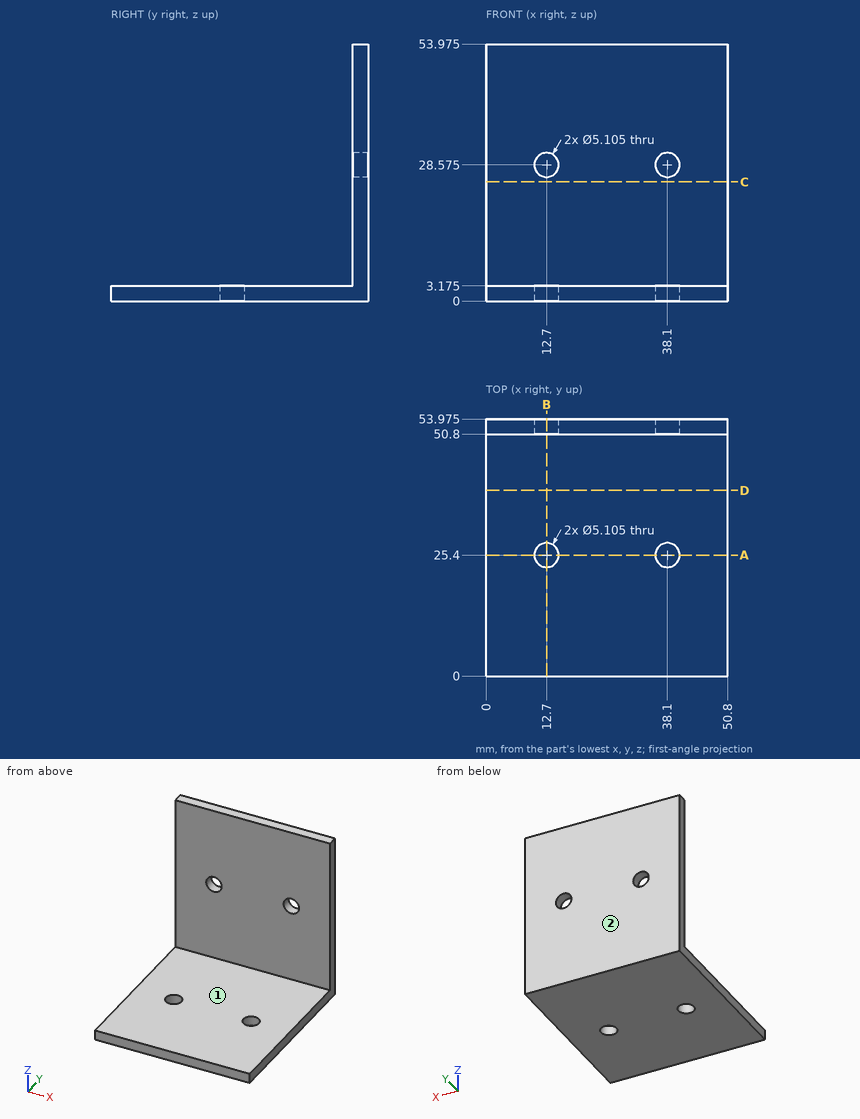
Input: dimensioned drawing with shaded views. Units: mm. Origin: part minimum x, y, z. A direction names the side the tool comes from. Round coordinates to 2 decimals unless told otherwise and drop trailing zeros. Order: outer loops, then holes, each group sorted by start corner. A loop starts at its lowest first (then second) coordinate and runs counter-clockwise, first axis right, second up. Notation, with made-up numbers: (24.5, -18.5) - (39.5, -18.5) arc R32 ccw to (39.5, 12.5) - close; hole circle Ø6 at (29, 48). An arc over 180 degrees is marked (long way). Answer as a JSON object with one key per item and string values. Group by question number.
(1) Pin query (flat end, axial travel): P1, Ø10, axis at x = 21.5, z = 27.5, coming from the -Y side. Return the tip coordinate at first contact, or that it passes through.
(2) Material intervals for probe 1 along Y at (x, z) = (38.1, 2.05) (1 decimal); probe 2 along Z at (x, y) = (38, 51) (1 decimal); probe 3 along Y at (x, z) = (24, 8) (1 decimal), sorted ascending. Write a range as from..to.
(3) Cut plane D-D (y = 39). Return loops of the section in (x, z) (1 decimal).
(4) Cut plane B-B (x = 12.7). Return loops of the section in (y, z) (1 decimal), then the cut area to 3 significant figures.
(5) Cut plane A-A (y = 25.4). Return loops of the section in (x, z) (1 decimal).
(6) Cut plane C-C (z = 25). Return loops of the section in (x, y) (1 decimal).
(7) Reachability of the marked faces 1 and 2 from +Z, -Z, +X, -X, +Y, -Y: full face, straight path, thin tool, end or side. Return the list, or none.
Here are the results:
{
 "1": {"P1": "stops at y = 50.8"},
 "2": {"probe 1": "y = 0..22.8, 28..54", "probe 2": "z = 0..26, 31.1..54", "probe 3": "y = 50.8..54"},
 "3": {"outline": "(0, 0) - (50.8, 0) - (50.8, 3.2) - (0, 3.2) - close"},
 "4": {"outline": "(0, 0) - (22.8, 0) - (22.8, 3.2) - (0, 3.2) - close; (28, 0) - (54, 0) - (54, 26) - (50.8, 26) - (50.8, 3.2) - (28, 3.2) - close; (50.8, 31.1) - (54, 31.1) - (54, 54) - (50.8, 54) - close", "area": "300 mm^2"},
 "5": {"outline": "(0, 0) - (10.1, 0) - (10.1, 3.2) - (0, 3.2) - close; (15.3, 0) - (35.5, 0) - (35.5, 3.2) - (15.3, 3.2) - close; (40.7, 0) - (50.8, 0) - (50.8, 3.2) - (40.7, 3.2) - close"},
 "6": {"outline": "(0, 50.8) - (50.8, 50.8) - (50.8, 54) - (0, 54) - close"},
 "7": {"face 1": "+Z, +X, -X, -Y", "face 2": "+Z, -Z, +X, -X, +Y"}
}
